Part model, mm, in its own coordinate system. Round coordinates to 2 decimals unless told otherwise and drop trailing zeros. Write each loop counter-clockwise with the first axis right and the second up, starting at its lowest first coordinate (ties: lowest second). Pieces come first, ordered by that corner, then holes. Notation, with made-up numbers: M -12.5,23.5 L 30.5,23.5 A24 ccw 30.5,45.5 Z; hole C -27.5,-7.75 d7. An arc over 180 degrees is marked long. Use a Markdown table: item, result. Add a question column.
1) Wall check: probe 1 along Z at (x, y) = (-18.5, 18.5); probe 2 along Z at (x, y) = (11.5, 32.5); probe 3 along X at (y, z) = (26.5, -16.5). Give the ranges that are in metal, low to high.
2) Slice it at A-A on y = 16.5. Write the cut outline in (x, z), plus the area to 3 significant figures.
3) Slice it at B-B on x = -12. Write the cut outline in (y, z), plus the area to 3 significant figures.
4) Slice it at C-C on z = -30. Write the cut outline in (x, y), plus the area to 3 significant figures.
5) Drop flat-ended pins along their axis: P1, Ø5, axis at x = 13, y = 17, coming from the +Z side; P2, Ø8, axis at x = -10.5, z = 17, coming from the -Y side; P3, Ø6, axis at x = 20.5, y = 19.5, coming from the +Z side. Give the stop position or say it passes through.
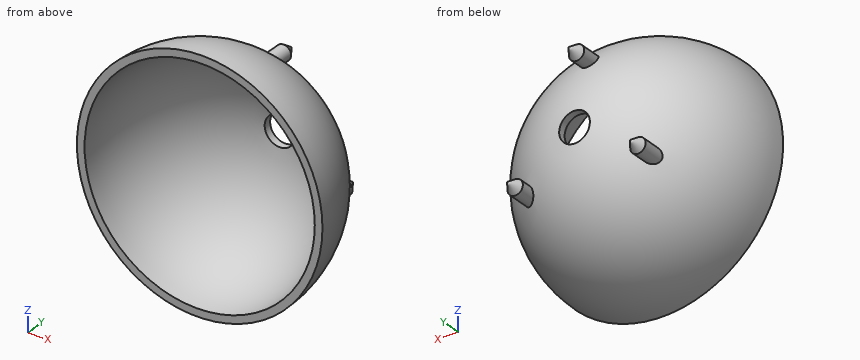
```python
from build123d import *

# Parameters (mm, degrees)
EXTRUDE1_REACH    = 41.37
SKETCH2_R         = 2.54
SKETCH4_R         = 5.08
EXTRUDE3_DEPTH    = 41.64
CIRPATTERN1_COUNT = 3


with BuildPart() as part:
    # Sketch1 → Revolve1 (revolve)
    with BuildSketch(Plane.XY):
        with BuildLine():
            Line((38.1, 0), (40.64, 0))
            ThreePointArc((40.64, 0), (28.736819587, 28.736819587), (0, 40.64))
            Line((0, 40.64), (0, 38.1))
            ThreePointArc((0, 38.1), (26.940768363, 26.940768363), (38.1, 0))
        make_face()
    revolve(axis=Axis((0, 38.1, 0), (0, 1, 0)))

    # Sketch2 → Extrude1 (add, up to next)
    with BuildSketch(Plane.XZ.offset(-39.37), mode=Mode.PRIVATE) as extrude1_sk1:
        with Locations((0, 23.46351494)):
            Circle(SKETCH2_R)
    extrude1_tool1 = extrude(extrude1_sk1.sketch, amount=EXTRUDE1_REACH, mode=Mode.PRIVATE) - part.part
    add(extrude1_tool1.solids().sort_by_distance((0, 39.37, 23.463515))[0])
    # Sketch2 → Extrude1 (add, up to next)
    with BuildSketch(Plane.XZ.offset(-39.37), mode=Mode.PRIVATE) as extrude1_sk2:
        with Locations((-20.32, -11.73175747)):
            Circle(SKETCH2_R)
    extrude1_tool2 = extrude(extrude1_sk2.sketch, amount=EXTRUDE1_REACH, mode=Mode.PRIVATE) - part.part
    add(extrude1_tool2.solids().sort_by_distance((-20.32, 39.37, -11.731757))[0])
    # Sketch2 → Extrude1 (add, up to next)
    with BuildSketch(Plane.XZ.offset(-39.37), mode=Mode.PRIVATE) as extrude1_sk3:
        with Locations((20.32, -11.73175747)):
            Circle(SKETCH2_R)
    extrude1_tool3 = extrude(extrude1_sk3.sketch, amount=EXTRUDE1_REACH, mode=Mode.PRIVATE) - part.part
    add(extrude1_tool3.solids().sort_by_distance((20.32, 39.37, -11.731757))[0])

    # Sketch4 → Extrude3 (cut, through all)
    with BuildSketch(Plane.XZ):
        Circle(SKETCH4_R)
    extrude(amount=-EXTRUDE3_DEPTH, mode=Mode.SUBTRACT)

    # Sketch5 → Revolve2 (revolve)
    with BuildSketch(Plane(origin=(0, 0, 0), x_dir=(0, 0, -1), z_dir=(1, 0, 0))):
        Polygon((-20.92351494, 39.37), (-23.46351494, 43.18), (-23.46351494, 39.37), align=None)
    revolve2 = revolve(axis=Axis((0, 39.37, 23.46351494), (0, 1, 0)))

    # CirPattern1: Revolve2 ×3 about axis
    cirpattern1_axis = Axis((0, 0, 0), (0, 1, 0))
    for i in range(1, CIRPATTERN1_COUNT):
        add(revolve2.rotate(cirpattern1_axis, i * 360 / CIRPATTERN1_COUNT))


solid = part.part
```
Entries:
| question | item | result |
|---|---|---|
| 1 | probe 1 | z = -31.1 to -27.7, 27.7 to 31.1 |
| 1 | probe 2 | z = -21.52 to -16.22, 16.22 to 21.52 |
| 1 | probe 3 | x = -26.02 to -21.84, 21.84 to 26.02 |
| 2 | outline | C 0,0 d74.28; hole C 0,0 d68.68 |
| 2 | area | 628 mm^2 |
| 3 | outline | M 0,-38.83 A38.83 ccw 0,38.83 L 0,36.16 A36.16 cw 0,-36.16 Z |
| 3 | area | 314 mm^2 |
| 4 | outline | M -27.42,0 L -23.49,0 A23.49 cw 23.49,0 L 27.42,0 A27.42 ccw Z |
| 4 | area | 314 mm^2 |
| 5 | P1 | stops at z = 35.98 |
| 5 | P2 | stops at y = 29.61 |
| 5 | P3 | stops at z = 31.81 |
